from build123d import *

# Parameters (mm, degrees)
F2_DEPTH = 500
F3_DEPTH = 250
F5_D     = 6
F5_DEPTH = 12


with BuildPart() as f2:
    # F1 (on Top) → F2 (new body, symmetric)
    with BuildSketch(Plane.XY):
        with BuildLine():
            Line((0, 0), (5, 0))
            Line((5, 0), (5, 250))
            ThreePointArc((5, 250), (3.477591, 257.653669), (-0.857864, 264.142136))
            Line((-0.857864, 264.142136), (-177.63456, 440.918831))
            Line((-177.63456, 440.918831), (-181.170094, 437.383297))
            Line((-181.170094, 437.383297), (-4.393398, 260.606602))
            ThreePointArc((-4.393398, 260.606602), (-1.141807, 255.740251), (0, 250))
            Line((0, 250), (0, 0))
        make_face()
    extrude(amount=F2_DEPTH, both=True)

    # F0 (on Right) → F3 (intersect, symmetric)
    with BuildSketch(Plane.YZ):
        Polygon((800, -184.694553), (0, 0), (0, -250), (800, -434.694553), align=None)
    extrude(amount=F3_DEPTH, both=True, mode=Mode.INTERSECT)

    # F5
    with Locations(Plane(origin=(131.642136, 131.642136, 0), x_dir=(-0.707107, 0.707107, 0), z_dir=(0.707107, 0.707107, 0))):
        with Locations((208.493665, -122.293395), (233.493665, -122.293395), (258.493665, -122.293395), (283.493665, -122.293395), (308.493665, -122.293395), (208.493665, -147.293395), (308.493665, -147.293395), (258.493665, -172.293395), (258.493665, -147.293395), (258.493665, -297.293395), (308.493665, -247.293395), (208.493665, -172.293395), (208.493665, -197.293395), (208.493665, -247.293395), (208.493665, -297.293395), (308.493665, -272.293395), (258.493665, -222.293395), (383.493665, -122.293395), (258.493665, -272.293395), (333.493665, -197.293395), (358.493665, -272.293395), (308.493665, -197.293395), (258.493665, -197.293395), (283.493665, -147.293395), (283.493665, -222.293395), (233.493665, -222.293395), (333.493665, -172.293395), (283.493665, -172.293395), (233.493665, -272.293395), (258.493665, -247.293395), (383.493665, -297.293395), (283.493665, -297.293395), (333.493665, -297.293395), (233.493665, -297.293395), (383.493665, -172.293395), (383.493665, -247.293395), (383.493665, -147.293395), (333.493665, -247.293395), (308.493665, -172.293395), (333.493665, -147.293395), (283.493665, -247.293395), (233.493665, -247.293395), (358.493665, -247.293395), (383.493665, -272.293395), (283.493665, -272.293395), (333.493665, -272.293395), (358.493665, -197.293395), (383.493665, -222.293395), (233.493665, -147.293395), (333.493665, -222.293395), (308.493665, -297.293395), (233.493665, -172.293395), (233.493665, -197.293395), (358.493665, -147.293395), (358.493665, -222.293395), (283.493665, -197.293395), (358.493665, -172.293395), (383.493665, -197.293395), (308.493665, -222.293395), (208.493665, -272.293395), (358.493665, -297.293395), (208.493665, -222.293395), (358.493665, -122.293395), (333.493665, -122.293395)):
            Hole(F5_D / 2, depth=F5_DEPTH)


solid = f2.part
Could you check a few things on this model? Use its own coordinates, in mm. A direction names the side the tool comes from. Coordinates: 2 decimals unless noted, no trailing zeros. Order: outer loops, then holes, each group sorted by start corner. A loop starts at its lowest first (then second) coordinate and runs counter-clockwise, first axis right, second up. Notation, with made-up numbers: (61, 49) -> (106, 49) arc R13 cw to (106, 73) -> close; hole circle Ø2 at (-16, 34.5). An arc over 180 degrees is marked (long way). One line per item, written item: value. Start each with the question number.
1) Imagine slicing it at D-D on y = 339. List the corners of the cut face in (x, z) for me.
2) Imagine slicing it at B-B on z = -71. List the corners of the cut face in (x, y) for me, plus the area to 3 significant figures.
3) Which directions (+Z, -Z, +X, -X, +Y, -Y) give clear straight access to the entire face, cutting with the end or side of a thin tool? Please do faces 1 (the flat face through (1.99, 219.43, -300.66)), 2 (the flat face through (0, 127, -152)).
4) I'm going to push flat-ended pins straight in: pin 1 (8 mm diameter, centred on x = -86, z = -296, fed in from +Y); pin 2 (1.5 mm diameter, centred on y = 348.5, z = -223, fed in from -X); pin 3 (5 mm diameter, centred on y = 396, z = -154.5, fed in from -X). Where does each tip first touch, or does it pass through?
5) Imagine slicing it at C-C on y = 213. List the corners of the cut face in (x, z) for me.
6) If I drill on L1, parallel to X at y = 29, z = -196.5; L2, parallel to X at y = 412, z = -163.5; L3, parallel to Y at x = -13.5, z = -207, over which ranges is the centre line in solid material (lowest first)? Write a range as [from, to].
7) Imagine slicing it at A-A on z = -108. List the corners of the cut face in (x, y) for me, plus the area to 3 significant figures.
Answer list:
1. outline: (-82.79, -328.26) -> (-75.72, -328.26) -> (-75.72, -78.26) -> (-82.79, -78.26) -> close
2. outline: (-51.32, 307.53) -> (-4.39, 260.61) arc R15 cw to (0, 250) -> (0, 0) -> (5, 0) -> (5, 250) arc R20 ccw to (-0.86, 264.14) -> (-44.25, 307.53) -> close
2. area: 1,640 mm2
3. face 1: -Z, +X, -X, -Y
3. face 2: +Z, -Z, -X, -Y
4. pin 1: stops at y = 353.28
4. pin 2: stops at x = -93.04
4. pin 3: stops at x = -142.29
5. outline: (0, -299.17) -> (5, -299.17) -> (5, -49.17) -> (0, -49.17) -> close
6. L1: x = [0, 5]
6. L2: x = [-155.79, -148.72]
6. L3: y = [269.71, 276.78]
7. outline: (-181.17, 437.38) -> (-4.39, 260.61) arc R15 cw to (0, 250) -> (0, 0) -> (5, 0) -> (5, 250) arc R20 ccw to (-0.86, 264.14) -> (-177.63, 440.92) -> close
7. area: 2,570 mm2
